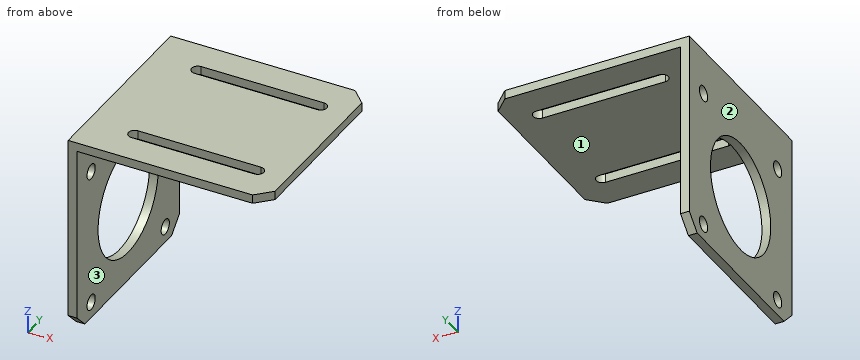
```python
from build123d import *

# Parameters (mm, degrees)
EXTRUDE_1_DEPTH     = 65
SKETCH_2_R          = 19.1
SKETCH_2_R_2        = 2.6
CUT_EXTRUDE_1_DEPTH = 117.073252733
CUT_EXTRUDE_2_DEPTH = 115.341593482
CHAMFER_1_SIZE      = 5


with BuildPart() as part:
    # 草图1 → 凸台-拉伸1 (new body)
    with BuildSketch(Plane(origin=(0, 0, 0), x_dir=(1, 0, 0), z_dir=(0, 1, 0))):
        Polygon((0, 0), (68, 0), (68, 3), (3, 3), (3, 68), (0, 68), align=None)
    extrude(amount=EXTRUDE_1_DEPTH)

    # 草图2 → 切除-拉伸1 (cut, through all)
    with BuildSketch(Plane.ZY):
        with Locations((-39, 32.5)):
            Circle(SKETCH_2_R)
        with Locations((-62.5, 56)):
            Circle(SKETCH_2_R_2)
        with Locations((-62.5, 9)):
            Circle(SKETCH_2_R_2)
        with Locations((-15.5, 56)):
            Circle(SKETCH_2_R_2)
        with Locations((-15.5, 9)):
            Circle(SKETCH_2_R_2)
    extrude(amount=-CUT_EXTRUDE_1_DEPTH, mode=Mode.SUBTRACT)

    # 草图3 → 切除-拉伸2 (cut, through all)
    with BuildSketch(Plane(origin=(0, 0, -3), x_dir=(-1, 0, 0), z_dir=(0, 0, -1))):
        with BuildLine():
            Line((-16, 14.6), (-58, 14.6))
            ThreePointArc((-58, 14.6), (-60.1, 12.5), (-58, 10.4))
            Line((-58, 10.4), (-16, 10.4))
            ThreePointArc((-16, 10.4), (-13.9, 12.5), (-16, 14.6))
        make_face()
    cut_extrude_2 = extrude(amount=-CUT_EXTRUDE_2_DEPTH, mode=Mode.SUBTRACT)

    # 镜向1: 切除-拉伸2 across plane
    add(cut_extrude_2.mirror(Plane.ZX.offset(32.5)), mode=Mode.SUBTRACT)

    # 倒角1
    chamfer_1_edges = [part.edges().sort_by_distance(p)[0] for p in [
        (1.5, 65, -68),
        (68, 65, -1.5),
        (68, 0, -1.5),
        (1.5, 0, -68),
    ]]
    chamfer(chamfer_1_edges, length=CHAMFER_1_SIZE)


solid = part.part
```
Read the model definition and answer for the solid it produces. Units are mm, in the model's axes. Face numbers are marked on the shaded views. Give positions to 0.01 mm unless a question says otherwise; leave off trailing zeros. Loops run counter-clockwise (first coordinate to the right, second up) from the corner with the lowest first, then second, coordinate; pieces in that order, holes last.
Item 1: The part is cut by section A-A (z = -15.5). Write down the section's boundary in (x, y), and give its area (3 significant figures).
Item 2: Find the intervals of material crossed by line 1 along Y through (x, z) = (1.35, -15.5); line 2 along X through (y, z) = (44, -22.5); line 3 along Z through (x, y) = (52, 33.5), in increasing order.
Item 3: The mould has two halves that part along X. Classify the marked faces 1, 2 and 3: released by +X, released by -X, zero draft, split by the parting line, or undercut.
Item 4: The part is cut by section D-D (y = 29). Write down the section's boundary in (x, z).
Item 5: Each of these flat-tipped pins is pushed along its axis until it touches: pin 1 Ø8.5 at (y, z) = (56, -15.5) entering from +X; pin 2 Ø6 at (x, y) = (52, 52) entering from +Z. Where does it stop, or does it pass through?
Item 6: The part is cut by section C-C (z = -39). Write down the section's boundary in (x, y), and give its area (3 significant figures).
Item 7: The part is cut by section B-B (x = 49). Write down the section's boundary in (y, z), and give its area (3 significant figures).
Taken from the geometry:
1. outline: (0, 0) - (3, 0) - (3, 6.4) - (0, 6.4) - close; (0, 11.6) - (3, 11.6) - (3, 53.4) - (0, 53.4) - close; (0, 58.6) - (3, 58.6) - (3, 65) - (0, 65) - close
1. area: 164 mm2
2. line 1: y = 0 to 6.4, 11.6 to 53.4, 58.6 to 65
2. line 2: x = 0 to 3
2. line 3: z = -3 to 0
3. face 1: zero draft
3. face 2: released by -X
3. face 3: released by +X
4. outline: (0, -68) - (3, -68) - (3, -57.78) - (0, -57.78) - close; (0, -20.22) - (3, -20.22) - (3, -3) - (68, -3) - (68, 0) - (0, 0) - close
5. pin 1: stops at x = 3
5. pin 2: stops at z = 0
6. outline: (0, 0) - (3, 0) - (3, 13.4) - (0, 13.4) - close; (0, 51.6) - (3, 51.6) - (3, 65) - (0, 65) - close
6. area: 80.4 mm2
7. outline: (0, -3) - (10.4, -3) - (10.4, 0) - (0, 0) - close; (14.6, -3) - (50.4, -3) - (50.4, 0) - (14.6, 0) - close; (54.6, -3) - (65, -3) - (65, 0) - (54.6, 0) - close
7. area: 170 mm2
